Geometry: final body of the model. Coordinates: model frame, mm. Face numbers are marked on the shaded views. A direction names the side the tool comes from. Round coordinates to 2 decimals unless told otherwise and drop trailing zeros. Order: outer loops, then holes, each group sorted by start corner. A loop starts at its lowest first (then second) coordinate and runs counter-clockwise, first axis right, second up. Notation, with made-up numbers: (2.5, 64) -> (35.5, 64) arc R27 ccw to (35.5, 83) -> close; hole circle Ø6 at (19.5, -24.75). An arc over 180 degrees is marked (long way). Put each result on its own line as item: value.
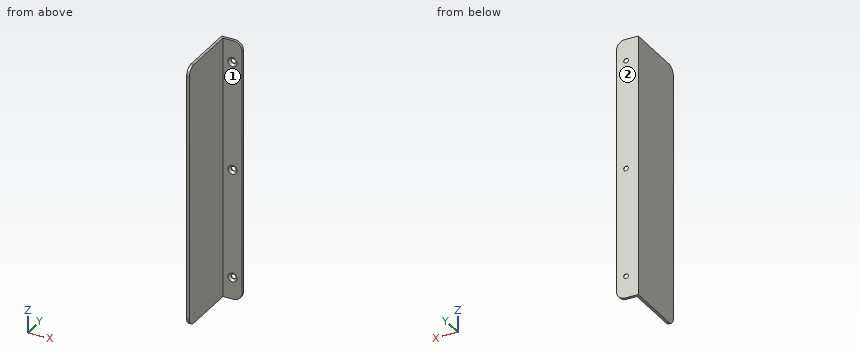
```python
from build123d import *

# Parameters (mm, degrees)
EXTRUDE_THIN1_DEPTH                            = 152.4
CSK_FOR_M5_FLAT_HEAD_MACHINE_SCREW1_AT_2_COUNT = 2
CSK_FOR_M5_FLAT_HEAD_MACHINE_SCREW1_AT_2_PITCH = 127
CSK_FOR_M5_FLAT_HEAD_MACHINE_SCREW1_AT_3_COUNT = 2
CSK_FOR_M5_FLAT_HEAD_MACHINE_SCREW1_AT_3_PITCH = 254
FILLET1_R                                      = 10


with BuildPart() as part:
    # Sketch1 → Extrude-Thin1 (new, symmetric)
    with BuildSketch(Plane.XY):
        Polygon((0, 0), (-25.4, 0), (-25.4, -76.2), (-22.225, -76.2), (-22.225, -3.175), (0, -3.175), align=None)
    extrude(amount=EXTRUDE_THIN1_DEPTH, both=True)

    # Sketch3 → CSK for M5 Flat Head Machine Screw1 (revolve, cut)
    with BuildSketch(Plane(origin=(-11.1125, -3.175, 127), x_dir=(0, 0, -1), z_dir=(1, 0, 0))):
        Polygon((0, 0), (0, 3.175), (2.75, 3.175), (2.75, 2.45), (5.2, 0), align=None)
    csk_for_m5_flat_head_machine_screw1 = revolve(axis=Axis((-11.1125, -9.525, 127), (0, 1, 0)), mode=Mode.SUBTRACT)

    # CSK for M5 Flat Head Machine Screw1 at 2: CSK for M5 Flat Head Machine Screw1 ×2
    with Locations(*[(0, 0, -i * CSK_FOR_M5_FLAT_HEAD_MACHINE_SCREW1_AT_2_PITCH) for i in range(1, CSK_FOR_M5_FLAT_HEAD_MACHINE_SCREW1_AT_2_COUNT)]):
        add(csk_for_m5_flat_head_machine_screw1, mode=Mode.SUBTRACT)

    # CSK for M5 Flat Head Machine Screw1 at 3: CSK for M5 Flat Head Machine Screw1 ×2
    with Locations(*[(0, 0, -i * CSK_FOR_M5_FLAT_HEAD_MACHINE_SCREW1_AT_3_PITCH) for i in range(1, CSK_FOR_M5_FLAT_HEAD_MACHINE_SCREW1_AT_3_COUNT)]):
        add(csk_for_m5_flat_head_machine_screw1, mode=Mode.SUBTRACT)

    # Fillet1
    fillet1_edges = [part.edges().sort_by_distance(p)[0] for p in [
        (0, -1.5875, 152.4),
        (0, -1.5875, -152.4),
        (-23.8125, -76.2, -152.4),
        (-23.8125, -76.2, 152.4),
    ]]
    fillet(fillet1_edges, radius=FILLET1_R)


solid = part.part
```
1. Cut plane C-C on y = -59. Return loops of the section in (x, z) (3 decimals).
Ans:
outline: (-25.4, -152.4) -> (-22.225, -152.4) -> (-22.225, 152.4) -> (-25.4, 152.4) -> close
2. Set-up query: the marked faces 1 and 2. Return all of +Z, -Z, +X, -X, +Y, -Y with unobstructed straight access to the full face (end or side cutting, diameter ignored); none if empty.
Ans:
face 1: +Z, -Z, +X, -Y
face 2: +Z, -Z, +X, -X, +Y
3. Cut plane D-D on x = -3. Return loops of the section in (y, z) (3 decimals).
Ans:
outline: (-3.175, -149.541) -> (0, -149.541) -> (0, 149.541) -> (-3.175, 149.541) -> close
4. Cut plane B-B on z = 11. Return loops of the section in (x, y) (3 decimals).
Ans:
outline: (-25.4, -76.2) -> (-22.225, -76.2) -> (-22.225, -3.175) -> (0, -3.175) -> (0, 0) -> (-25.4, 0) -> close
5. Material intervals for probe 1 along X at (y, z) = (-0.25, -127); probe 2 along X at (y, z) = (-69, -120.5) (3 decimals); probe 3 along Y at (x, z) = (-18.25, -115) (3 decimals), sorted ascending.
Ans:
probe 1: -25.4 to -13.86, -8.36 to 0
probe 2: -25.4 to -22.225
probe 3: -3.175 to 0
6. Contact query for flat-ended pins moving along their axis: P1, Ø9, axis at x = -11.11, z = -127, coming from the +Y side; P2, Ø1.5, axis at y = -51.5, z = -48.5, coming from the +X side (3 decimals); P3, Ø5, axis at x = -16, z = -46.5, coming from the -Y side (3 decimals). Output: stop coordinate, or through.
Ans:
P1: y = 0
P2: x = -22.225
P3: y = -3.175
7. Cut plane A-A on z = -127. Return loops of the section in (x, y) (1 decimal).
Ans:
outline: (-25.4, -76.2) -> (-22.2, -76.2) -> (-22.2, -3.2) -> (-16.3, -3.2) -> (-13.9, -0.7) -> (-13.9, 0) -> (-25.4, 0) -> close; (-8.4, -0.7) -> (-5.9, -3.2) -> (0, -3.2) -> (0, 0) -> (-8.4, 0) -> close
